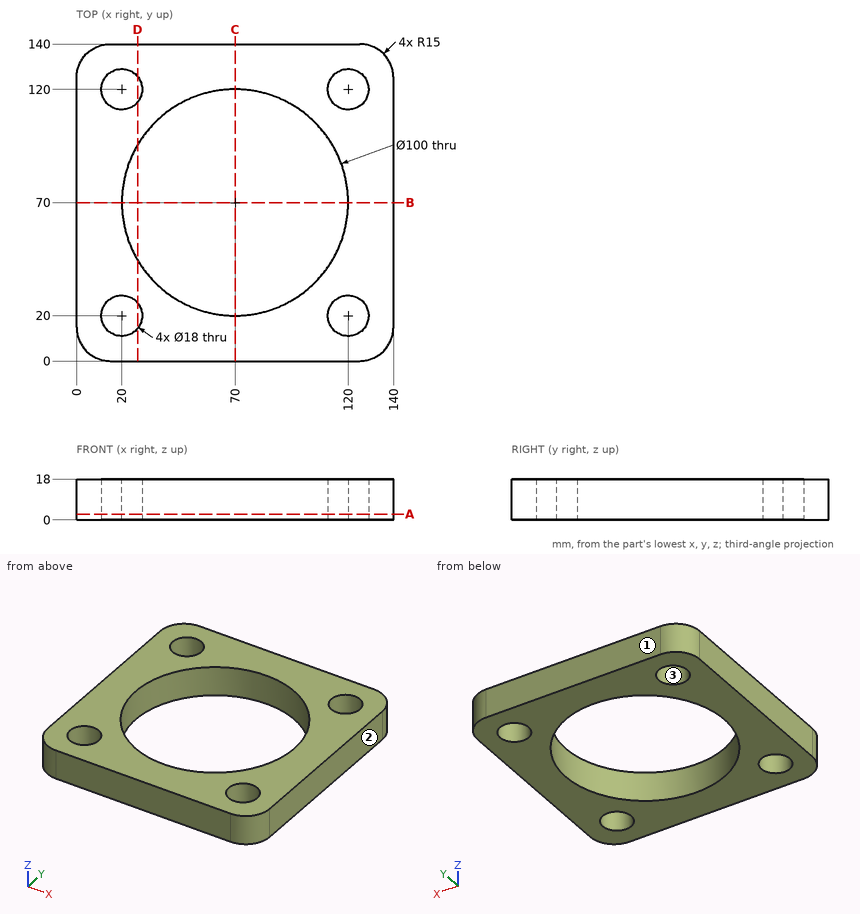
Input: dimensioned drawing with shaded views. Units: mm. Origin: part minimum x, y, z. Coordinates: 2 decimals unless noted, no trailing zeros. Loops run counter-clockwise (first coordinate to the right, second up) from the corner with the lowest first, then second, coordinate; pieces in that order, holes last. Notation, with made-up numbers: M -2.5,43.5 L 54.5,43.5 A17 ccw 54.5,56.5 Z; hole C 46,-10.5 d8. An arc over 180 degrees is marked long. Put each result on its own line as item: value.
(1) Cut plane A-A on z = 2.5. Return the cut outline in (x, y).
Answer sheet:
outline: M 0,15 A15 ccw 15,0 L 125,0 A15 ccw 140,15 L 140,125 A15 ccw 125,140 L 15,140 A15 ccw 0,125 Z; hole C 20,20 d18; hole C 20,120 d18; hole C 70,70 d100; hole C 120,20 d18; hole C 120,120 d18
(2) Material intervals for probe 1 along Y at (x, z) = (70, 4); probe 2 along X at (y, z) = (115, 13); probe 3 along Y at (x, z) = (91.5, 7.5), sorted ascending.
Answer sheet:
probe 1: y = 0 to 20, 120 to 140
probe 2: x = 0 to 12.52, 27.48 to 48.21, 91.79 to 112.52, 127.48 to 140
probe 3: y = 0 to 24.86, 115.14 to 140
(3) Draft query along Y for the marked faces 1, 2 and 3. Return one class per face: pulls with the +Y half, pulls with the -Y half, needs draft (parallel to the pull), parting line crosses it, or undercut.
Answer sheet:
face 1: pulls with the +Y half
face 2: needs draft
face 3: undercut
(4) Cut plane B-B on y = 70. Return the cut outline in (x, z), then the cut area to 3 significant figures.
Answer sheet:
outline: M 0,0 L 20,0 L 20,18 L 0,18 Z; M 120,0 L 140,0 L 140,18 L 120,18 Z
area: 720 mm^2
(5) Cut plane D-D on x = 27. Return the cut outline in (y, z).
Answer sheet:
outline: M 0,0 L 14.34,0 L 14.34,18 L 0,18 Z; M 25.66,0 L 44.49,0 L 44.49,18 L 25.66,18 Z; M 95.51,0 L 114.34,0 L 114.34,18 L 95.51,18 Z; M 125.66,0 L 140,0 L 140,18 L 125.66,18 Z
